```python
from build123d import *

# Parameters (mm, degrees)
SALIENTE_EXTRUIR1_DEPTH = 920


with BuildPart() as part:
    # Croquis1 → Saliente-Extruir1 (new body)
    with BuildSketch(Plane(origin=(0, 0, 0), x_dir=(1, 0, 0), z_dir=(0, 1, 0))):
        with BuildLine():
            Line((-27.04570475, 0.111036701), (-27.04570475, -0.9709854))
            ThreePointArc((-27.04570475, -0.9709854), (-27.106772974, -1.136359948), (-27.260665216, -1.222355571))
            ThreePointArc((-27.260665216, -1.222355571), (-27.673358623, -1.810535113), (-27.070917054, -2.202115474))
            Line((-27.070917054, -2.202115474), (-26.38570475, -2.202115474))
            ThreePointArc((-26.38570475, -2.202115474), (-26.173572716, -2.114247508), (-26.08570475, -1.902115474))
            Line((-26.08570475, -1.902115474), (-26.08570475, 0.111036701))
            ThreePointArc((-26.08570475, 0.111036701), (-26.092347771, 0.237887611), (-26.112204161, 0.36335078))
            ThreePointArc((-26.112204161, 0.36335078), (-26.06688189, 0.594292482), (-25.868853352, 0.721465107))
            ThreePointArc((-25.868853352, 0.721465107), (-19.52570475, 1.480091061), (-13.182556148, 0.721465107))
            ThreePointArc((-13.182556148, 0.721465107), (-12.984527611, 0.594292482), (-12.93920534, 0.36335078))
            ThreePointArc((-12.93920534, 0.36335078), (-12.959061729, 0.237887611), (-12.96570475, 0.111036701))
            Line((-12.96570475, 0.111036701), (-12.96570475, -1.902115474))
            ThreePointArc((-12.96570475, -1.902115474), (-12.877836785, -2.114247508), (-12.66570475, -2.202115474))
            Line((-12.66570475, -2.202115474), (-11.980492447, -2.202115474))
            ThreePointArc((-11.980492447, -2.202115474), (-11.378050878, -1.810535113), (-11.790744285, -1.222355571))
            ThreePointArc((-11.790744285, -1.222355571), (-11.944636526, -1.136359948), (-12.00570475, -0.9709854))
            Line((-12.00570475, -0.9709854), (-12.00570475, 0.111036701))
            ThreePointArc((-12.00570475, 0.111036701), (-11.943640246, 0.277569223), (-11.787723385, 0.362862925))
            ThreePointArc((-11.787723385, 0.362862925), (-11.352050184, 0.596107617), (-11.166986384, 1.054327667))
            ThreePointArc((-11.166986384, 1.054327667), (-11.230212618, 1.249640519), (-11.40422216, 1.358568688))
            ThreePointArc((-11.40422216, 1.358568688), (-19.52570475, 2.441214001), (-27.64718734, 1.358568688))
            ThreePointArc((-27.64718734, 1.358568688), (-27.821196883, 1.249640519), (-27.884423117, 1.054327667))
            ThreePointArc((-27.884423117, 1.054327667), (-27.699359317, 0.596107617), (-27.263686116, 0.362862925))
            ThreePointArc((-27.263686116, 0.362862925), (-27.107769254, 0.277569223), (-27.04570475, 0.111036701))
        make_face()
    extrude(amount=SALIENTE_EXTRUIR1_DEPTH)


solid = part.part
```
CAD build for the part. Positions are in the model's coordinates, mm. Round coordinates to 2 decimals unless told otherwise and drop trailing zeros. Write each loop counter-clockwise with the first axis right and the second up, starting at its lowest first coordinate (ties: lowest second). Pieces come first, ordered by that corner, then holes. Notation, with made-up numbers: M 78,-33 L 132,-33 A12 cw 132,-25 Z; hole C 2,78 d2. An arc over 180 degrees is marked long. One line per question, with ' | ' between items.
1. Pin check, flat tips, straight feed: pin 1 Ø1.5 at (y, z) = (451, 0) entering from +X; pin 2 Ø1.5 at (x, y) = (-18.5, 768) entering from -Z; pin 3 Ø0.5 at (y, z) = (281, 0.5) entering from -X. Stop position of each tip, or through.
Working result:
pin 1: x = -11.25 | pin 2: z = -2.44 | pin 3: x = -27.05
2. Cut at A-A on y = 695.5. Write the cut outline in (x, z).
Working result:
outline: M -27.88,-1.05 A0.3 ccw -27.65,-1.36 A31 ccw -11.4,-1.36 A0.3 ccw -11.17,-1.05 A0.73 ccw -11.79,-0.36 A0.25 cw -12.01,-0.11 L -12.01,0.97 A0.25 cw -11.79,1.22 A0.5 ccw long -11.98,2.2 L -12.67,2.2 A0.3 ccw -12.97,1.9 L -12.97,-0.11 A1.21 ccw -12.94,-0.36 A0.3 cw -13.18,-0.72 A26.9 cw -25.87,-0.72 A0.3 cw -26.11,-0.36 A1.21 ccw -26.09,-0.11 L -26.09,1.9 A0.3 ccw -26.39,2.2 L -27.07,2.2 A0.5 ccw long -27.26,1.22 A0.25 cw -27.05,0.97 L -27.05,-0.11 A0.25 cw -27.26,-0.36 A0.73 ccw Z
3. Probe L1, parallel to X at y = 416, z = 0.25; L2, parallel to X at y = 582.5, z = 1.95; L3, parallel to Z at x = -21, y = 136.5. List the from-to ranges inside material, lowest first. Write a range as from..to.
Working result:
L1: -27.05..-26.09, -12.97..-12.01 | L2: -27.62..-26.09, -12.96..-11.43 | L3: -2.41..-1.44
4. Cut at B-B on x = -21. Write the cut outline in (y, z), and give its area (3 significant figures).
Working result:
outline: M 0,-2.41 L 920,-2.41 L 920,-1.44 L 0,-1.44 Z | area: 889 mm2
